Geometry: final body of the model. Coordinates: model frame, mm. A direction names the side the tool comes from. Round coordinates to 2 decimals unless told otherwise and drop trailing zeros. Loops run counter-clockwise (first coordinate to the right, second up) from the corner with the lowest first, then second, coordinate; pieces in that order, holes last. Notation, with made-up numbers: M 20,-19.75 L 42,-19.75 A19 ccw 42,13.25 Z; hole C -2.5,-34 d6. An arc over 180 degrees is marked long. Write each question's results on one line, items separated by ' | '.
```python
from build123d import *

# Parameters (mm, degrees)
SKETCH1_R                                           = 11.5
BOSS_EXTRUDE1_DEPTH                                 = 5.5
CUT_EXTRUDE1_START                                  = 2
SKETCH1_3_R                                         = 12.65
CUT_EXTRUDE1_DEPTH                                  = 3.5
CBORE_FOR_M3_HEX_SOCKET_HEAD_CAP_SCREW1_D           = 3.4
CBORE_FOR_M3_HEX_SOCKET_HEAD_CAP_SCREW1_DEPTH       = 45
CBORE_FOR_M3_HEX_SOCKET_HEAD_CAP_SCREW1_CBORE_D     = 6.5
CBORE_FOR_M3_HEX_SOCKET_HEAD_CAP_SCREW1_CBORE_DEPTH = 3.4
CBORE_FOR_M3_HEX_SOCKET_HEAD_CAP_SCREW1_TIP         = 1.021463052


with BuildPart() as part:
    # Sketch1 → Boss-Extrude1 (new body)
    with BuildSketch(Plane(origin=(0, 0, 0), x_dir=(1, 0, 0), z_dir=(0, 1, 0))):
        with BuildLine():
            ThreePointArc((-4, -22), (0, -26), (4, -22))
            Line((4, -22), (4, -17.549928775))
            ThreePointArc((4, -17.549928775), (15.588457268, -9), (17.198684154, 5.310862772))
            Line((17.198684154, 5.310862772), (21.052558883, 7.535898385))
            ThreePointArc((21.052558883, 7.535898385), (22.516660498, 13), (17.052558883, 14.464101615))
            Line((17.052558883, 14.464101615), (13.198684154, 12.239066003))
            ThreePointArc((13.198684154, 12.239066003), (0, 18), (-13.198684154, 12.239066003))
            Line((-13.198684154, 12.239066003), (-17.052558883, 14.464101615))
            ThreePointArc((-17.052558883, 14.464101615), (-22.516660498, 13), (-21.052558883, 7.535898385))
            Line((-21.052558883, 7.535898385), (-17.198684154, 5.310862772))
            ThreePointArc((-17.198684154, 5.310862772), (-15.588457268, -9), (-4, -17.549928775))
            Line((-4, -17.549928775), (-4, -22))
        make_face()
        Circle(SKETCH1_R, mode=Mode.SUBTRACT)
    extrude(amount=BOSS_EXTRUDE1_DEPTH)

    # Sketch1<3> → Cut-Extrude1 (cut)
    with BuildSketch(Plane(origin=(0, 0, 0), x_dir=(1, 0, 0), z_dir=(0, 1, 0)).offset(CUT_EXTRUDE1_START)):
        Circle(SKETCH1_3_R)
    extrude(amount=CUT_EXTRUDE1_DEPTH, mode=Mode.SUBTRACT)

    # CBORE for M3 Hex Socket Head Cap Screw1
    with Locations(Plane.XZ):
        with Locations((-19.052558883, -11), (19.052558883, -11), (0, 22)):
            CounterBoreHole(CBORE_FOR_M3_HEX_SOCKET_HEAD_CAP_SCREW1_D / 2, CBORE_FOR_M3_HEX_SOCKET_HEAD_CAP_SCREW1_CBORE_D / 2, CBORE_FOR_M3_HEX_SOCKET_HEAD_CAP_SCREW1_CBORE_DEPTH, depth=CBORE_FOR_M3_HEX_SOCKET_HEAD_CAP_SCREW1_DEPTH)
            with Locations((0, 0, -(CBORE_FOR_M3_HEX_SOCKET_HEAD_CAP_SCREW1_DEPTH + CBORE_FOR_M3_HEX_SOCKET_HEAD_CAP_SCREW1_TIP / 2))):  # 118° drill point
                Cone(0, CBORE_FOR_M3_HEX_SOCKET_HEAD_CAP_SCREW1_D / 2, CBORE_FOR_M3_HEX_SOCKET_HEAD_CAP_SCREW1_TIP, mode=Mode.SUBTRACT)


solid = part.part
```
1. Section B-B (y = 4). Output: boundary loops of the cut face in (x, z), then the cut area to 3 significant figures.
Answer key:
outline: M -21.05,-7.54 A4 ccw -17.05,-14.46 L -13.2,-12.24 A18 ccw 13.2,-12.24 L 17.05,-14.46 A4 ccw 21.05,-7.54 L 17.2,-5.31 A18 ccw 4,17.55 L 4,22 A4 ccw -4,22 L -4,17.55 A18 ccw -17.2,-5.31 Z; hole C -19.05,-11 d3.4; hole C 0,0 d25.3; hole C 0,22 d3.4; hole C 19.05,-11 d3.4 | area: 663 mm²
2. Draft query along X for faces 4 (the face through (-15.7, 2.7, 8.8)), 5 (the face through (-5, 0, -11)), 6 (the face through (-1.5, 1, -11.4)), 7 (the face through (19.1, 2.71, -6.41)). Return one class per face: pulls with the +X half, pulls with the -X half, needs draft (parallel to the pull), parting line crosses it, or undercut.
Answer key:
face 4: pulls with the -X half | face 5: needs draft | face 6: undercut | face 7: pulls with the +X half
3. Access query for faces 1 (the face through (15.153, 2.712, -13.367)), 2 (the face through (-17.7, 3.4, -12.4)), 3 (the face through (4, 3, 20)). Directions: +Z, -Z, +X, -X, +Y, -Y. A direction counts if a zero-diameter tool reaches every point of the face in a straight line with its end or side. Return the directions, or none.
Answer key:
face 1: -Z, +Y, -Y | face 2: -Y | face 3: +Z, +X, +Y, -Y
4. Ray query, probe 1 along Z at (x, y) = (0, 2.65); probe 2 along Z at (x, y) = (0, 1.05); probe 3 along X at (y, z) = (3, 0). Return the intervals inside material, ascending.
Answer key:
probe 1: z = -18 to -12.65, 12.65 to 18.75, 25.25 to 26 | probe 2: z = -18 to -11.5, 11.5 to 18.75, 25.25 to 26 | probe 3: x = -18 to -12.65, 12.65 to 18
5. Section D-D (z = 10.5). Output: boundary loops of the cut face in (x, y), then the cut area to 3 significant figures.
Answer key:
outline: M -14.62,0 L -4.69,0 L -4.69,2 L -7.05,2 L -7.05,5.5 L -14.62,5.5 Z; M 4.69,0 L 14.62,0 L 14.62,5.5 L 7.05,5.5 L 7.05,2 L 4.69,2 Z | area: 92.7 mm²
6. Pin query (flat end, axial travel): P1, Ø1.5, axis at x = -11, y = 3.5, coming from the +Z side; P2, Ø1, axis at y = 3.5, z = -3, coming from the +X side; P3, Ø6, axis at x = 0, z = 22, coming from the -Y side. Return the tip coordinate at first contact, or that it passes through.
Answer key:
P1: stops at z = 14.8 | P2: stops at x = 17.83 | P3: stops at y = 3.4
7. Section A-A (x = 0). Output: boundary loops of the cut face in (y, z).
Answer key:
outline: M 0,-18 L 5.5,-18 L 5.5,-12.65 L 2,-12.65 L 2,-11.5 L 0,-11.5 Z; M 0,11.5 L 2,11.5 L 2,12.65 L 5.5,12.65 L 5.5,20.3 L 3.4,20.3 L 3.4,18.75 L 0,18.75 Z; M 0,25.25 L 3.4,25.25 L 3.4,23.7 L 5.5,23.7 L 5.5,26 L 0,26 Z
8. Section C-C (x = -7). Output: boundary loops of the cut face in (y, z).
Answer key:
outline: M 0,-16.58 L 5.5,-16.58 L 5.5,-10.54 L 2,-10.54 L 2,-9.12 L 0,-9.12 Z; M 0,9.12 L 2,9.12 L 2,10.54 L 5.5,10.54 L 5.5,16.58 L 0,16.58 Z
